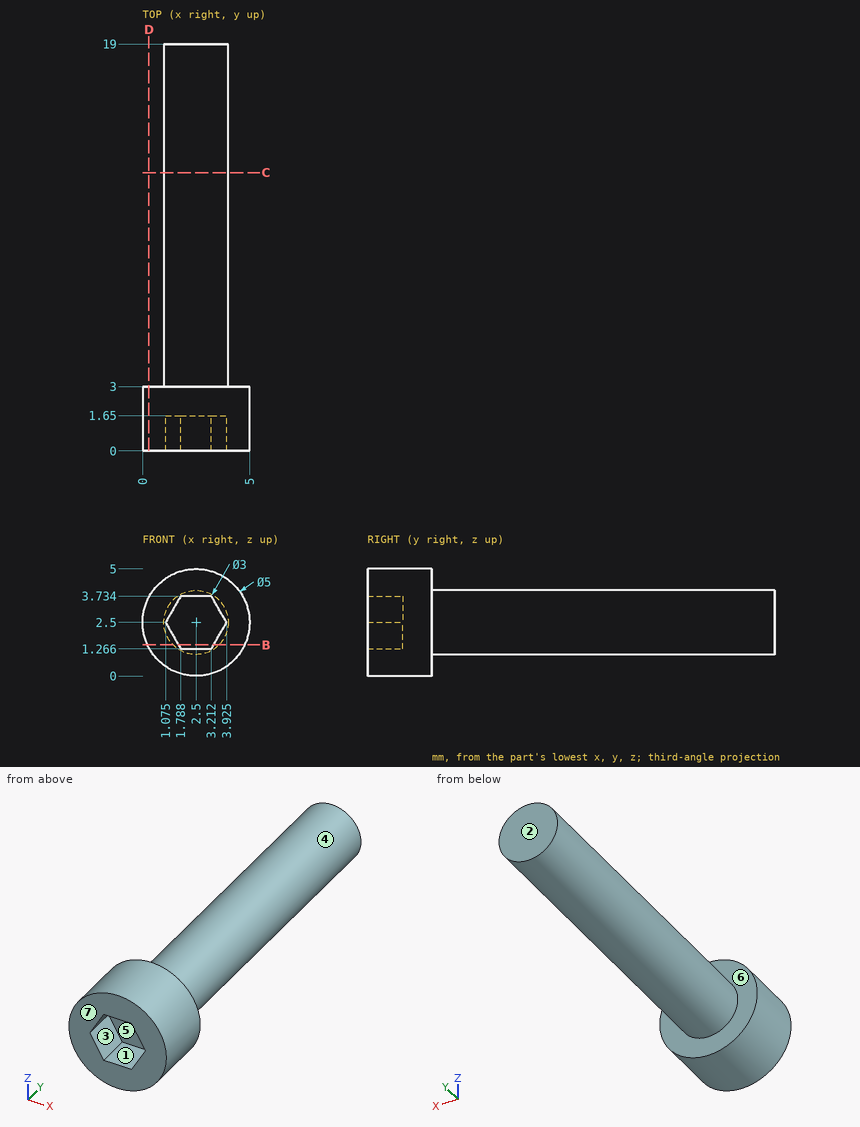
Drawing for the job (mm, zero at the part's lowest x, y, z). A direction names the side the tool comes from. Round coordinates to 2 decimals unless told otherwise and drop trailing zeros. Write each loop counter-clockwise with the first axis right and the second up, starting at its lowest first coordinate (ties: lowest second). Pieces come first, ordered by that corner, then holes. Notation, with made-up numbers: (-21.5, 25.25) - (-8.5, 25.25) arc R5 cw to (-8.5, 31.25) - close; hole circle Ø11 at (22, 37). An arc over 180 degrees is marked (long way). Write item = value, one per line. Start each with the question number.
Q1. Band-saw the part on C-C (y = 13). Give the cut face in (x, z).
Q2. Band-saw the part on D-D (x = 0.3). Give the cut face in (y, z).
Q3. Mould opens along Z. For the marked faces 1, 2, 3 and 4 say: pulls with the +Z half, pulls with the -Z half, needs draft (parallel to the pull), parting line crosses it, or undercut.
Q4. Which spindle directions (+Z, -Z, +X, -X, +Y, -Y) get a long thin tool onto all of the face, cutting with end or side? Do the marked faces 5, 6 and 7. Say none if no direction does.
Q5. Probe L1, parallel to Y at x = 0.55, z = 3.3; L2, parallel to Y at x = 2.4, z = 2.15; L3, parallel to Z at x = 2.7, y = 15. List the from-to ranges inside material, lowest first. Write a range as from..to.
Q6. Band-saw the part on B-B (z = 1.45). Give the cut face in (x, y).
Q7. Drop flat-ended pins along their axis: pin 1 (1.2 mm diameter, centred on x = 2.5, z = 2, fed in from -Y); pin 2 (3 mm diameter, centred on x = 1.5, y = 8, fed in from -Z); pin 3 (0.7 mm diameter, centred on x = 3, y = 0.5, fed in from +Z) (1 decimal). Give the stop position or say it passes through.
Answers below:
q1.outline = circle Ø3 at (2.5, 2.5)
q2.outline = (0, 1.31) - (3, 1.31) - (3, 3.69) - (0, 3.69) - close
q3.face_1 = undercut
q3.face_2 = needs draft
q3.face_3 = undercut
q3.face_4 = parting line crosses it
q4.face_5 = -Y
q4.face_6 = +Y
q4.face_7 = +Z, -Z, +X, -X, -Y
q5.L1 = 0..3
q5.L2 = 1.65..19
q5.L3 = 1.01..3.99
q6.outline = (0.23, 0) - (1.68, 0) - (1.68, 1.65) - (3.32, 1.65) - (3.32, 0) - (4.77, 0) - (4.77, 3) - (3.57, 3) - (3.57, 19) - (1.43, 19) - (1.43, 3) - (0.23, 3) - close
q7.pin_1 = 1.65
q7.pin_2 = 1
q7.pin_3 = 5
